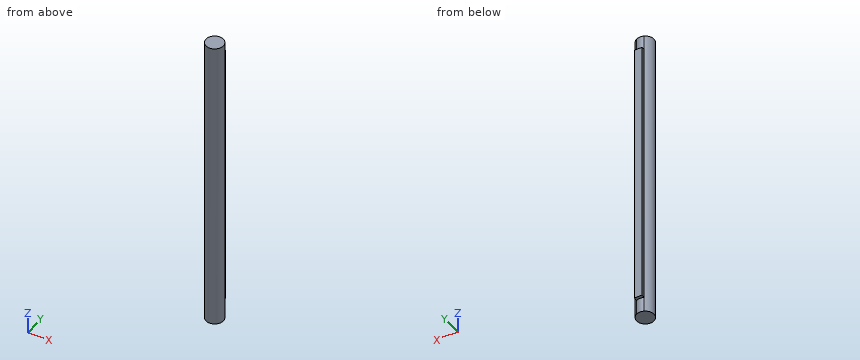
```python
from build123d import *

# Parameters (mm, degrees)
BOSS_EXTRU_1_DEPTH      = 121
ENL_V_START             = -6
ENL_V_MAT_EXTRU_1_DEPTH = 6
ENL_V_MAT_EXTRU_2_DEPTH = 6


with BuildPart() as part:
    # Esquisse1 → Boss.-Extru.1 (new body)
    with BuildSketch(Plane.XY):
        with BuildLine():
            Line((-1.5, 3.16227766), (-1.5, 4.66227766))
            Line((-1.5, 4.66227766), (1.5, 4.66227766))
            Line((1.5, 4.66227766), (1.5, 3.16227766))
            ThreePointArc((1.5, 3.16227766), (0, -3.5), (-1.5, 3.16227766))
        make_face()
    extrude(amount=BOSS_EXTRU_1_DEPTH)

    # Esquisse2 → Enlèv. mat.-Extru.1 (cut)
    with BuildSketch(Plane.XY.offset(121).offset(ENL_V_START)):
        with BuildLine():
            ThreePointArc((-1.5, 3.16227766), (0, 3.5), (1.5, 3.16227766))
            Line((1.5, 3.16227766), (1.5, 4.66227766))
            Line((1.5, 4.66227766), (-1.5, 4.66227766))
            Line((-1.5, 4.66227766), (-1.5, 3.16227766))
        make_face()
    extrude(amount=ENL_V_MAT_EXTRU_1_DEPTH, mode=Mode.SUBTRACT)

    # Esquisse3 → Enlèv. mat.-Extru.2 (cut)
    with BuildSketch(Plane(origin=(0, 0, 0), x_dir=(-1, 0, 0), z_dir=(0, 0, -1))):
        with BuildLine():
            Line((-1.5, 4.66227766), (-1.5, 3.16227766))
            ThreePointArc((-1.5, 3.16227766), (0, 3.5), (1.5, 3.16227766))
            Line((1.5, 3.16227766), (1.5, 4.66227766))
            Line((1.5, 4.66227766), (-1.5, 4.66227766))
        make_face()
    extrude(amount=-ENL_V_MAT_EXTRU_2_DEPTH, mode=Mode.SUBTRACT)


solid = part.part
```
Geometry check sheet. Reference: the model listing, model coordinates, mm. Coordinates: 2 decimals unless noted, no trailing zeros. Order: outer loops, then holes, each group sorted by start corner. A loop starts at its lowest first (then second) coordinate and runs counter-clockwise, first axis right, second up. Notation, with made-up numbers: (-33.5, 54.25) - (17.5, 54.25) arc R11 ccw to (17.5, 62.25) - close; hole circle Ø9 at (-25, 56). An arc over 180 degrees is marked (long way). Answer in a Markdown table with one row per item. Add a question column.
1. Section check C-C (y = -1.25). Enter the section's corners in (x, z), plus the area to 3 significant figures.
2. Section check B-B (z = 106.5). Enter the section's corners in (x, y), plus the area to 3 significant figures.
3. Gauge pin test, flat ends, axial feed: pin 1 Ø1 at (x, z) = (1, 17.5) entering from -Y; pin 2 Ø1.5 at (y, z) = (-1, 37.5) entering from -X; pin 3 Ø1 at (x, y) = (-1, 3.5) entering from -Z; pin 4 Ø1.2 at (y, z) = (4.5, 74.5) entering from +X. Record the tip position at first contact, or that the pin passes through.
4. Section check A-A (x = -0.5). Enter the section's corners in (y, z).
5. Material ranges on L1, parallel to X at y = -0.25, z = 76; L2, parallel to X at y = 3.75, z = 30; L3, parallel to Y at x = -1.75, z = 87.5, recorded low to high. Write a range as [from, to].
Data:
| question | item | result |
|---|---|---|
| 1 | outline | (-3.27, 0) - (3.27, 0) - (3.27, 121) - (-3.27, 121) - close |
| 1 | area | 791 mm² |
| 2 | outline | (-1.5, 3.16) arc R3.5 ccw (long way) to (1.5, 3.16) - (1.5, 4.66) - (-1.5, 4.66) - close |
| 2 | area | 42.3 mm² |
| 3 | pin 1 | stops at y = -3.46 |
| 3 | pin 2 | stops at x = -3.49 |
| 3 | pin 3 | stops at z = 0 |
| 3 | pin 4 | stops at x = 1.5 |
| 4 | outline | (-3.46, 0) - (3.46, 0) - (3.46, 6) - (4.66, 6) - (4.66, 115) - (3.46, 115) - (3.46, 121) - (-3.46, 121) - close |
| 5 | L1 | x = [-3.49, 3.49] |
| 5 | L2 | x = [-1.5, 1.5] |
| 5 | L3 | y = [-3.03, 3.03] |
